Autodesk Inventor part; units mm, degrees
ref_plane "YZ Plane" through (0, 0, 0) normal (1, 0, 0) x (0, 1, 0)
ref_plane "XZ Plane" through (0, 0, 0) normal (0, 1, 0) x (-1, 0, 0)
ref_plane "XY Plane" through (0, 0, 0) normal (0, 0, 1) x (1, 0, 0)
sketch "Sketch1" plane through (0, 0, 0) normal (0, 0, 1) x (1, 0, 0)
  line L0 (-14.65, 5.75) -> (-10.15, 5.75)
  line L1 (-10.15, 5.75) -> (-6.05, 1.65)
  line L2 (-6.05, 1.65) -> (6.05, 1.65)
  line L3 (6.05, 1.65) -> (10.15, 5.75)
  line L4 (10.15, 5.75) -> (14.65, 5.75)
  line L5 (-14.65, 5.75) -> (-14.65, -1.85)
  line L6 (-14.65, -1.85) -> (-8.15, -1.85)
  line L7 (-8.15, -1.85) -> (-8.15, -5.75)
  line L8 (-8.15, -5.75) -> (8.15, -5.75)
  line L9 (8.15, -5.75) -> (8.15, -1.85)
  line L10 (8.15, -1.85) -> (14.65, -1.85)
  line L11 (14.65, -1.85) -> (14.65, 5.75)
  line L12 (0, -5.75) -> (0, 5.75) construction
  point P0 (0, 0)
  point P1 (0, 0)
  dimension "d0" = 12.1
  dimension "d1" = 4.5
  dimension "d2" = 135
  dimension "d3" = 7.6
  dimension "d4" = 6.5
  dimension "d6" = 4.1
  dimension "d29" = 11.5
extrude "Extrusion1" add sketch "Sketch1" along normal mid plane 50
sketch "Sketch2" plane through (-14.65, 5.75, 25) normal (0, 1, 0) x (1, 0, 0)
  circle A0 centre (2.65, 34) radius 1.75
  line L0 (-5.86, 25) -> (35.16, 25)
  line L1 (14.65, 60) -> (14.65, -10)
  circle A1 centre (26.65, 34) radius 1.75
  circle A2 centre (2.65, 16) radius 1.75
  circle A3 centre (26.65, 16) radius 1.75
  line L2 (2.65, 16) -> (26.65, 16) construction
  line L3 (26.65, 16) -> (26.65, 34) construction
  line L4 (26.65, 34) -> (2.65, 34) construction
  line L5 (2.65, 34) -> (2.65, 16) construction
  point P0 (14.65, 25)
  point P1 (2.65, 25)
  point P2 (14.65, 34)
  dimension "d11" = 24
  dimension "d14" = 18
  dimension "d17" = 3.5
extrude "Extrusion2" cut sketch "Sketch2" against normal through all
sketch "Sketch3" plane through (-6.05, 1.65, 25) normal (0, 1, 0) x (1, 0, 0)
  circle A0 centre (6.05, 45) radius 2.75
  circle A1 centre (6.05, 5) radius 2.75
  line L0 (6.05, 5) -> (6.05, 45) construction
  line L1 (1.7705, 10) -> (10.3295, 10)
  line L2 (10.3295, 10) -> (10.3295, 40)
  line L3 (10.3295, 40) -> (1.7705, 40)
  line L4 (1.7705, 40) -> (1.7705, 10)
  line L5 (1.7705, 10) -> (10.3295, 40) construction
  line L6 (10.3295, 10) -> (1.7705, 40) construction
  circle A2 centre (6.05, 45) radius 4.25 construction
  point P0 (6.05, 25)
  point P1 (6.05, 25)
  dimension "d21" = 5.5
  dimension "d23" = 40
  dimension "d24" = 30
  dimension "d25" = 8.5
extrude "Extrusion3" cut sketch "Sketch3" against normal through all contours A0 | A1
fillet "Fillet2" radius 1 2 edges at (8.15, -1.85, 0) (-8.15, -1.85, 0)
properties part number "Acople_rodamiento_lineal"
The listing builds one solid part. Answer for the finished solid, in the listing's coordinates (mm). A direction names the side the tool comes from. Round coordinates to 2 decimals unless told otherwise and drop trailing zeros. Write each loop counter-clockwise with the first axis right and the second up, starting at its lowest first coordinate (ties: lowest second). Pieces come first, ordered by that corner, then holes. Notation, with made-up numbers: (48.5, 8.25) -> (107.5, 8.25) arc R35 cw to (107.5, 41.25) -> close; hole circle Ø8 at (-16, -29.75). An arc over 180 degrees is marked (long way). Answer as a JSON object with one key per item and string values. Group by question number.
Q1. Each of these flat-tipped pins is pushed along its axis until it touches: pin 1 Ø5.5 at (x, z) = (12, 9) entering from -Y; pin 2 Ø5 at (x, z) = (0, -20) entering from -Y; pin 3 Ø13.5 at (x, z) = (-1.5, -3) entering from +Y; pin 4 Ø8 at (x, z) = (1.5, -4.5) entering from +Y. Where does it stop, or does it pass through?
Q2. Section D-D (z = 9) is taken. Write down the section's boundary in (x, y), plus the area to 3 significant figures.
Q3. Determine the mould class of faces 5 (the face through (-0.358, -1.998, -22.727)), 6 (the face through (12, -1.85, 0)), 7 (the face through (0, 0, 25)), 8 (the face through (12.9, 2, 7.5)) for opening direction Z: pulls with the +Z half, pulls with the -Z half, needs draft (parallel to the pull), parting line crosses it, or undercut.
Q4. Section C-C (x = 0) is taken. Write down the section's boundary in (y, z).
Q5. Section A-A (y = 4) is taken. Write down the section's boundary in (x, z).
Q6. Section B-B (z = -20) is taken. Write down the section's boundary in (x, y), plus the area to 3 significant figures.
Q7. Straight lines are drawn through the part: line 1 along Z through (x, y) = (0, -2.5); line 2 along Z through (x, y) = (12, 0.5); line 3 along X through (y, z) = (-3.5, -20). For each, find the intervals that lie inside material, in ascending order.
Q8. Which of the six approach directions +Z, -Z, +X, -X, +Y, -Y give full straight-line access (tool end or side, diameter ignored) to faces 1 (the face through (8.1, 3.7, -0.4)), 2 (the face through (8.15, -4, 0)), 3 (the face through (-12, -1.85, 0)), 4 (the face through (14.65, 2, 0))?
Check values:
{
 "1": {"pin 1": "y = -1.85", "pin 2": "through", "pin 3": "y = 3.85", "pin 4": "y = 1.65"},
 "2": {"outline": "(-14.65, -1.85) -> (-13.75, -1.85) -> (-13.75, 5.75) -> (-14.65, 5.75) -> close; (-10.25, -1.85) -> (-9.15, -1.85) arc R1 cw to (-8.15, -2.85) -> (-8.15, -5.75) -> (8.15, -5.75) -> (8.15, -2.85) arc R1 cw to (9.15, -1.85) -> (10.25, -1.85) -> (10.25, 5.75) -> (10.15, 5.75) -> (6.05, 1.65) -> (-6.05, 1.65) -> (-10.15, 5.75) -> (-10.25, 5.75) -> close; (13.75, -1.85) -> (14.65, -1.85) -> (14.65, 5.75) -> (13.75, 5.75) -> close", "area": "167 mm^2"},
 "3": {"face 5": "undercut", "face 6": "needs draft", "face 7": "pulls with the +Z half", "face 8": "undercut"},
 "4": {"outline": "(-5.75, -25) -> (1.65, -25) -> (1.65, -22.75) -> (-5.75, -22.75) -> close; (-5.75, -17.25) -> (1.65, -17.25) -> (1.65, 17.25) -> (-5.75, 17.25) -> close; (-5.75, 22.75) -> (1.65, 22.75) -> (1.65, 25) -> (-5.75, 25) -> close"},
 "5": {"outline": "(-14.65, -25) -> (-8.4, -25) -> (-8.4, 25) -> (-14.65, 25) -> close; (8.4, -25) -> (14.65, -25) -> (14.65, 25) -> (8.4, 25) -> close; hole circle Ø3.5 at (-12, -9); hole circle Ø3.5 at (-12, 9); hole circle Ø3.5 at (12, -9); hole circle Ø3.5 at (12, 9)"},
 "6": {"outline": "(-14.65, -1.85) -> (-9.15, -1.85) arc R1 cw to (-8.15, -2.85) -> (-8.15, -5.75) -> (-2.75, -5.75) -> (-2.75, 1.65) -> (-6.05, 1.65) -> (-10.15, 5.75) -> (-14.65, 5.75) -> close; (2.75, -5.75) -> (8.15, -5.75) -> (8.15, -2.85) arc R1 cw to (9.15, -1.85) -> (14.65, -1.85) -> (14.65, 5.75) -> (10.15, 5.75) -> (6.05, 1.65) -> (2.75, 1.65) -> close", "area": "180 mm^2"},
 "7": {"line 1": "-25 to -22.75, -17.25 to 17.25, 22.75 to 25", "line 2": "-25 to -10.75, -7.25 to 7.25, 10.75 to 25", "line 3": "-8.15 to -2.75, 2.75 to 8.15"},
 "8": {"face 1": "+Z, -Z, +Y", "face 2": "+Z, -Z, +X, -Y", "face 3": "+Z, -Z, -X, -Y", "face 4": "+Z, -Z, +X, +Y, -Y"}
}
